from build123d import *

# Parameters (mm, degrees)
SKETCH1_W            = 211.1756
SKETCH1_H            = 127
BOSS_EXTRUDE1_DEPTH  = 6.35
M3_CLEARANCE_HOLE1_D = 3.4
SKETCH4_W            = 3.5052
SKETCH4_H            = 47.625
CUT_EXTRUDE1_DEPTH   = 247.50447569
CUT_EXTRUDE2_DEPTH   = 247.50447569
SKETCH6_W            = 121.4628
SKETCH6_H            = 6.35
CUT_EXTRUDE3_DEPTH   = 247.50447569


with BuildPart() as part:
    # Sketch1 → Boss-Extrude1 (new body)
    with BuildSketch(Plane.XY):
        with Locations((105.5878, 63.5)):
            Rectangle(SKETCH1_W, SKETCH1_H)
    extrude(amount=BOSS_EXTRUDE1_DEPTH)

    # M3 Clearance Hole1 (through all)
    with Locations(Plane.XY.offset(6.35)):
        with Locations((5.9944, 105.0036), (5.9944, 31.9786), (205.1812, 31.9786), (205.1812, 105.0036)):
            Hole(M3_CLEARANCE_HOLE1_D / 2)

    # Sketch4 → Cut-Extrude1 (cut, through all)
    with BuildSketch(Plane.XY.offset(6.35)):
        with Locations((48.7426, 84.1375)):
            Rectangle(SKETCH4_W, SKETCH4_H)
        with Locations((162.433, 84.1375)):
            Rectangle(SKETCH4_W, SKETCH4_H)
    extrude(amount=-CUT_EXTRUDE1_DEPTH, mode=Mode.SUBTRACT)

    # Sketch5 → Cut-Extrude2 (cut, through all)
    with BuildSketch(Plane.XY.offset(6.35)):
        Polygon((0, 12.608311795), (89.7128, 0), (0, 0), align=None)
        Polygon((121.4628, 0), (211.1756, 0), (211.1756, 12.608311795), align=None)
    extrude(amount=-CUT_EXTRUDE2_DEPTH, mode=Mode.SUBTRACT)

    # Sketch6 → Cut-Extrude3 (cut, through all)
    with BuildSketch(Plane.XY.offset(6.35)):
        with Locations((105.5878, 3.129155898)):
            Rectangle(SKETCH6_W, SKETCH6_H)
    extrude(amount=-CUT_EXTRUDE3_DEPTH, mode=Mode.SUBTRACT)


solid = part.part
Design review of the part built by this model. Coordinates are the model's own, in mm. A direction names the side the tool comes from. Round coordinates to 2 decimals unless told otherwise and drop trailing zeros. Write each loop counter-clockwise with the first axis right and the second up, starting at its lowest first coordinate (ties: lowest second). Pieces come first, ordered by that corner, then holes. Notation, with made-up numbers: (-33.75, 20.25) -> (22.25, 20.25) arc R17 cw to (22.25, 32.25) -> close; hole circle Ø1 at (-8, 63). An arc over 180 degrees is marked (long way). One line per item, written item: value. Start each with the question number.
Q1. Add section A-A (y = 95). Give the boundary of the cut face in (x, z), then the cut area to 3 significant figures.
Q2. Insertion check: P1, Ø1, axis at x = 27.5, z = 5.5, coming from the -Y side. The pin has a flat end and moves straight along its axis. Give the tip position at first contact, or say it passes through.
Q3. Tool access review of faces 1 (the face through (104, 67, 6.35)), 2 (the face through (50.495, 84, 3)): name each direction out of +Z, -Z, +X, -X, +Y, -Y from which nothing blocks a thin tool from reaching the whole face with its end or side.
Q4. The part is to be moulded in two halves that separate along Y. For faces 3 (the face through (160.68, 84, 3)), 4 (the face through (22.11, 9.5, 3.22)), 5 (the face through (211.176, 69, 3)), say which applies: pulls with the +Y half, pulls with the -Y half, needs draft (parallel to the pull), parting line crosses it, or undercut.
Q5. Add section D-D (x = 28). Give the boundary of the cut face in (y, z).
Q6. To check wall thickness, follow probe 1 along X at (y, z) = (69, 5.75); probe 2 along X at (y, z) = (33.5, 4.75); probe 3 along Y at (x, z) = (20.5, 1). State the ranges of each line that lie inside material, in increasing order.
Q7. Add section C-C (x = 192). Give the boundary of the cut face in (y, z).
Q8. Add section B-B (z = 4.75). Give the boundary of the cut face in (x, y) (3 decimals).
Response:
1. outline: (0, 0) -> (46.99, 0) -> (46.99, 6.35) -> (0, 6.35) -> close; (50.5, 0) -> (160.68, 0) -> (160.68, 6.35) -> (50.5, 6.35) -> close; (164.19, 0) -> (211.18, 0) -> (211.18, 6.35) -> (164.19, 6.35) -> close
1. area: 1,300 mm^2
2. P1: stops at y = 8.67
3. face 1: +Z, +X, -X, +Y, -Y
3. face 2: +Z, -Z
4. face 3: undercut
4. face 4: pulls with the -Y half
4. face 5: needs draft
5. outline: (8.67, 0) -> (127, 0) -> (127, 6.35) -> (8.67, 6.35) -> close
6. probe 1: x = 0 to 46.99, 50.5 to 160.68, 164.19 to 211.18
6. probe 2: x = 0 to 5.24, 6.75 to 204.42, 205.94 to 211.18
6. probe 3: y = 9.73 to 127
7. outline: (9.91, 0) -> (127, 0) -> (127, 6.35) -> (9.91, 6.35) -> close
8. outline: (0, 12.608) -> (44.856, 6.304) -> (166.319, 6.304) -> (211.176, 12.608) -> (211.176, 127) -> (0, 127) -> close; hole circle Ø3.4 at (5.994, 31.979); hole circle Ø3.4 at (5.994, 105.004); hole (46.99, 60.325) -> (50.495, 60.325) -> (50.495, 107.95) -> (46.99, 107.95) -> close; hole (160.68, 60.325) -> (164.186, 60.325) -> (164.186, 107.95) -> (160.68, 107.95) -> close; hole circle Ø3.4 at (205.181, 31.979); hole circle Ø3.4 at (205.181, 105.004)
